Here's how the part is built. I have some questions about the finished solid (model axes, mm). A direction names the side the tool comes from. Coordinates: 2 decimals unless noted, no trailing zeros. Order: outer loops, then holes, each group sorted by start corner. A loop starts at its lowest first (then second) coordinate and runs counter-clockwise, first axis right, second up.
```python
from build123d import *

# Parameters (mm, degrees)
SKETCH1_W           = 480
SKETCH1_H           = 511
SKETCH1_R           = 3
BOSS_EXTRUDE1_DEPTH = 15
SKETCH2_W           = 40
SKETCH2_H           = 40
SKETCH2_H_2         = 431
SKETCH2_W_2         = 440
CUT_EXTRUDE1_DEPTH  = 5
SKETCH3_R           = 100
CUT_EXTRUDE2_DEPTH  = 15
SKETCH4_R           = 1.5
CUT_EXTRUDE3_DEPTH  = 7
CUT_EXTRUDE4_DEPTH  = 2.3
SKETCH6_R           = 3
CUT_EXTRUDE5_DEPTH  = 7
SKETCH7_R           = 1.5
CUT_EXTRUDE6_DEPTH  = 5


with BuildPart() as part:
    # Sketch1 → Boss-Extrude1 (new body)
    with BuildSketch(Plane.XY):
        Rectangle(SKETCH1_W, SKETCH1_H)
        with Locations((-197, 240.5)):
            Circle(SKETCH1_R, mode=Mode.SUBTRACT)
        with Locations((-197, -235.5)):
            Circle(SKETCH1_R, mode=Mode.SUBTRACT)
        with Locations(Location((197, -235.5, 0), (0, 0, 180))):
            Circle(SKETCH1_R, mode=Mode.SUBTRACT)
        with Locations(Location((197, 240.5, 0), (0, 0, 180))):
            Circle(SKETCH1_R, mode=Mode.SUBTRACT)
    extrude(amount=BOSS_EXTRUDE1_DEPTH)

    # Sketch2 → Cut-Extrude1 (cut)
    with BuildSketch(Plane(origin=(0, 0, 0), x_dir=(-1, 0, 0), z_dir=(0, 0, -1))):
        Polygon((-200, 255.5), (-240, 255.5), (-240, 215.5), (200, 215.5), (200, 255.5), align=None)
        with Locations((220, 235.5)):
            Rectangle(SKETCH2_W, SKETCH2_H)
        with Locations((220, 0)):
            Rectangle(SKETCH2_W, SKETCH2_H_2)
        with Locations((-20, -235.5)):
            Rectangle(SKETCH2_W_2, SKETCH2_H)
        with Locations((220, -235.5)):
            Rectangle(SKETCH2_W, SKETCH2_H)
    extrude(amount=-CUT_EXTRUDE1_DEPTH, mode=Mode.SUBTRACT)

    # Sketch3 → Cut-Extrude2 (cut)
    with BuildSketch(Plane(origin=(0, 0, 0), x_dir=(-1, 0, 0), z_dir=(0, 0, -1))):
        Circle(SKETCH3_R)
    extrude(amount=-CUT_EXTRUDE2_DEPTH, mode=Mode.SUBTRACT)

    # Sketch4 → Cut-Extrude3 (cut)
    with BuildSketch(Plane(origin=(0, 0, 0), x_dir=(-1, 0, 0), z_dir=(0, 0, -1))):
        with Locations((22.80945209, 173.254989525)):
            Circle(SKETCH4_R)
        with Locations(Location((-22.80945209, 173.254989525, 0), (0, 0, 180))):
            Circle(SKETCH4_R)
        with Locations((-161.447948306, -66.873929806)):
            Circle(SKETCH4_R)
        with Locations(Location((-138.638496216, -106.381059719, 0), (0, 0, 180))):
            Circle(SKETCH4_R)
        with Locations((138.638496216, -106.381059719)):
            Circle(SKETCH4_R)
        with Locations(Location((161.447948306, -66.873929806, 0), (0, 0, 180))):
            Circle(SKETCH4_R)
    extrude(amount=-CUT_EXTRUDE3_DEPTH, mode=Mode.SUBTRACT)

    # Sketch5 → Cut-Extrude4 (cut)
    with BuildSketch(Plane(origin=(0, 0, 0), x_dir=(-1, 0, 0), z_dir=(0, 0, -1))):
        Polygon((22.80945209, 176.430416006), (20.05945209, 174.842702765), (20.05945209, 171.667276285), (22.80945209, 170.079563045), (25.55945209, 171.667276285), (25.55945209, 174.842702765), align=None)
        Polygon((-20.05945209, 174.842702765), (-20.05945209, 171.667276285), (-22.80945209, 170.079563045), (-25.55945209, 171.667276285), (-25.55945209, 174.842702765), (-22.80945209, 176.430416006), align=None)
        Polygon((-164.197948306, -68.461643046), (-161.447948306, -70.049356286), (-158.697948306, -68.461643046), (-158.697948306, -65.286216566), (-161.447948306, -63.698503325), (-164.197948306, -65.286216566), align=None)
        Polygon((-138.638496216, -109.5564862), (-141.388496216, -107.96877296), (-141.388496216, -104.793346479), (-138.638496216, -103.205633239), (-135.888496216, -104.793346479), (-135.888496216, -107.96877296), align=None)
        Polygon((141.388496216, -107.96877296), (141.388496216, -104.793346479), (138.638496216, -103.205633239), (135.888496216, -104.793346479), (135.888496216, -107.96877296), (138.638496216, -109.5564862), align=None)
        Polygon((164.197948306, -65.286216566), (164.197948306, -68.461643046), (161.447948306, -70.049356286), (158.697948306, -68.461643046), (158.697948306, -65.286216566), (161.447948306, -63.698503325), align=None)
    extrude(amount=-CUT_EXTRUDE4_DEPTH, mode=Mode.SUBTRACT)

    # Sketch6 → Cut-Extrude5 (cut)
    with BuildSketch(Plane(origin=(0, 0, 0), x_dir=(-1, 0, 0), z_dir=(0, 0, -1))):
        with Locations((-156.911542489, 135.010250847)):
            Circle(SKETCH6_R)
    extrude(amount=-CUT_EXTRUDE5_DEPTH, mode=Mode.SUBTRACT)

    # Sketch7 → Cut-Extrude6 (cut)
    with BuildSketch(Plane(origin=(0, 0, 0), x_dir=(-1, 0, 0), z_dir=(0, 0, -1))):
        with Locations((-123.323970382, 168.597822953)):
            Circle(SKETCH7_R)
        with Locations((-190.499114595, 168.597822953)):
            Circle(SKETCH7_R)
        with Locations((-190.499114595, 101.422678741)):
            Circle(SKETCH7_R)
    extrude(amount=-CUT_EXTRUDE6_DEPTH, mode=Mode.SUBTRACT)


solid = part.part
```
Q1. If we section it at D-D on y = 152: Write out the boundary of the cut face in (x, z).
Q2. Will these pins go through, and if not, where does the flat tip stop? pin 1 (1.5 mm diameter, centred on x = 184, z = 4, fed in from -Y); pin 2 (5.5 mm diameter, centred on y = -4, z = 1.5, fed in from -X); pin 3 (2.5 mm diameter, centred on x = -139, y = -106, fed in from -Z).
Q3. We'd pull the mould along Y, two halves only. Please class faces 1 (the flat face through (240, -4, 7)), 2 (the cylindrical face through (-95.38, 30.04, 7.4)): pulls with the +Y half, pulls with the -Y half, needs draft (parallel to the pull), parting line crosses it, or undercut.
Q4. If we section it at C-C on y = -18: Write out the boundary of the cut face in (x, z).
Q5. I need wall thicknesses on L1, parallel to Y at x = -197, z = 8.5; L2, parallel to X at y = 240.5, z = 8.5; L3, parallel to X at y = 2.5, z = 10.5. Which ranges of each line are inside material? Lowest first, please.
Q6. If we section it at B-B on z = 12.5: Write out the boundary of the cut face in (x, y).
Q7. If we section it at A-A on x = 0: Write out the boundary of the cut face in (y, z), then the cut area to 4 significant figures.
Q8. For faces 3 (the flat face through (-110, 4, 15)), 4 (the flat face through (-212, -37, 5)), which set-ups out of +Z, -Z, +X, -X, +Y, -Y let a thin tool reach every point of the face, with its end or its side?
Reply:
1. outline: (-240, 5) - (-200, 5) - (-200, 0) - (240, 0) - (240, 15) - (-240, 15) - close
2. pin 1: stops at y = -215.5
2. pin 2: stops at x = -200
2. pin 3: stops at z = 2.3
3. face 1: needs draft
3. face 2: undercut
4. outline: (-240, 5) - (-200, 5) - (-200, 0) - (-98.37, 0) - (-98.37, 15) - (-240, 15) - close; (98.37, 0) - (240, 0) - (240, 15) - (98.37, 15) - close
5. L1: y = -255.5 to -238.5, -232.5 to 237.5, 243.5 to 255.5
5. L2: x = -240 to -200, -194 to 194, 200 to 240
5. L3: x = -240 to -99.97, 99.97 to 240
6. outline: (-240, -255.5) - (240, -255.5) - (240, 255.5) - (-240, 255.5) - close; hole circle Ø6 at (-197, -235.5); hole circle Ø6 at (-197, 240.5); hole circle Ø200 at (0, 0); hole circle Ø6 at (197, -235.5); hole circle Ø6 at (197, 240.5)
7. outline: (-255.5, 5) - (-215.5, 5) - (-215.5, 0) - (-100, 0) - (-100, 15) - (-255.5, 15) - close; (100, 0) - (215.5, 0) - (215.5, 5) - (255.5, 5) - (255.5, 15) - (100, 15) - close
7. area: 4,265 mm2
8. face 3: +Z, +X, -X, +Y, -Y
8. face 4: -Z, -X
